Design review of the part built by this model. Coordinates are the model's own, in mm. Face numbers are marked on the shaded views. A direction names the side the tool comes from. Coordinates: 2 decimals unless noted, no trailing zeros. Write each loop counter-clockwise with the first axis right and the second up, starting at its lowest first coordinate (ties: lowest second). Pieces come first, ordered by that corner, then holes.
Q1. Insertion check: pin 1 (3 mm diameter, centred on x = -2, z = 25, fed in from +Y); pin 2 (12 mm diameter, centred on y = 17.5, z = 82, fed in from +X); pin 3 (4 mm diameter, centred on y = -12, z = 10, fed in from +X); pin 4 (2 mm diameter, centred on x = 28, y = 29.5, fed in from +Z). Each pin has a flat end and moves straight along its axis. Give the tip position at first contact, or say it passes through.
Q2. Take a section at A-A (z = 69). Give the boundary of the cut face in (x, y).
Q3. Take a section at B-B (y = 2). Give the boundary of the cut face in (x, z).
Q4. Machinability: for the marked faces 4, 5 and 6, which of the approach directions +Z, -Z, +X, -X, +Y, -Y give a long, thin tool a straight path to every point of the face, cutting with its end or side? Answer none if there is none.
Q5. Take a section at D-D (x = 33). Give the boundary of the cut face in (y, z), and give its area (3 significant figures).
Q6. Take a section at C-C (x = 15.5). Give the boundary of the cut face in (y, z), and give its area (3 significant figures).
Q7. Mouldability with a two-part tool opening along X and no side actions: class the marked faces 1, 2 and 3 as pulls with the +X half, pulls with the -X half, needs draft (parallel to the pull), parting line crosses it, or undercut.
Q8. For probe 1 along X at (y, z) = (1, 35); probe 2 along Z at (x, y) = (-25.5, 3.5); probe 3 along X at (y, z) = (5.5, 100.5), list the stretches that pass through material, from the lowest coordinate up.
Autodesk Fusion 360 part; units mm, degrees
sketch "Sketch1" plane through (0, 0, 0) normal (0, 0, 1) x (1, 0, 0)
  circle A0 centre (0, 0) radius 38.1
  circle A1 centre (0, 0) radius 37.1
  line L0 (24.903, -27.5) -> (24.903, 27.5)
  line L1 (26.903, -25.5468) -> (26.903, 25.5468)
  line L2 (26.903, 12.5) -> (28.903, 12.5)
  line L3 (28.903, 12.5) -> (28.903, -12.5)
  line L4 (28.903, -12.5) -> (26.903, -12.5)
  line L5 (26.903, -12.5) -> (26.903, 12.5)
  line L6 (26.903, 14.5) -> (30.903, 14.5)
  line L7 (30.903, 14.5) -> (30.903, 9.5)
  line L8 (30.903, 9.5) -> (28.903, 9.5)
  line L9 (26.903, -14.5) -> (30.903, -14.5)
  line L10 (30.903, -14.5) -> (30.903, -9.5)
  line L11 (30.903, -9.5) -> (28.903, -9.5)
  line L12 (1.75, 0) -> (22.5, 0)
  line L13 (24.903, 26.75) -> (22.903, 26.75)
  line L14 (22.903, 26.75) -> (22.903, -26.75)
  line L15 (22.903, -26.75) -> (24.903, -26.75)
  line L16 (24.903, -26.75) -> (24.903, 26.75)
  line L17 (22.903, 18.08) -> (11.903, 18.08)
  line L18 (11.903, 18.08) -> (11.903, 5.58)
  line L19 (11.903, 5.58) -> (22.903, 5.58)
  line L20 (22.903, 5.58) -> (22.903, 18.08)
  line L21 (22.903, -13.25) -> (11.903, -13.25)
  line L22 (11.903, -13.25) -> (11.903, -22.5)
  line L23 (11.903, -22.5) -> (22.903, -22.5)
  line L24 (22.903, -22.5) -> (22.903, -13.25)
  line L25 (30.903, -9.5) -> (30.903, 9.5)
  line L26 (0, -38.1) -> (0, 38.1) construction
  line L27 (-38.1, 0) -> (38.1, 0) construction
  line L28 (26.9408, -26.9408) -> (-26.9408, 26.9408) construction
  line L29 (26.9408, 26.9408) -> (-26.9408, -26.9408) construction
  line L30 (0, 37.1) -> (0, 38.1)
  line L31 (-26.2337, 26.2337) -> (-26.9408, 26.9408)
  line L32 (-37.1, 0) -> (-38.1, 0)
  line L33 (-26.9408, -26.9408) -> (-26.2337, -26.2337)
  line L34 (0, -38.1) -> (0, -37.1)
  line L35 (26.9408, -26.9408) -> (26.2337, -26.2337)
  line L36 (38.1, 0) -> (37.1, 0)
  line L37 (26.9408, 26.9408) -> (26.2337, 26.2337)
  line L38 (20.903, 30.6508) -> (20.903, 20.08)
  line L39 (20.903, 20.08) -> (9.903, 20.08)
  line L40 (9.903, 20.08) -> (9.903, 3.58)
  line L41 (9.903, 3.58) -> (22.903, 3.58)
  point P0 (28.903, 0)
  point P1 (22.903, 0)
  dimension "d1" = 76.2
  dimension "d2" = 1
  dimension "d3" = 55
  dimension "d4" = 2
  dimension "d5" = 2
  dimension "d6" = 2
  dimension "d7" = 2
  dimension "d8" = 3
  dimension "d9" = 25
  dimension "d10" = 2
  dimension "d11" = 2
  dimension "d12" = 53.5
  dimension "d13" = 12.5
  dimension "d14" = 11
  dimension "d15" = 8.67
  dimension "d16" = 9.25
  dimension "d17" = 11
  dimension "d18" = 4.25
  dimension "d23" = 45
  dimension "d27" = 2
  dimension "d28" = 2
  dimension "d29" = 2
  dimension "d30" = 2
extrude "Extrude1" add sketch "Sketch1" along normal blind 2 contours A1 L1 L6 L7 L9 L10 L25 | A1 L0 L14 L15 L21 L22 L23 L38 L39 L40 L41 | A1 L0 L13 L14 L17 L18 L19 L38 L39 L40 L41 | L0 L13 L14 L15 L16 L20 L24 makes body 1 at (-3.5853, -7.0522, 0) makes body 2 at (32.7043, -2.5435, 0)
extrude "Extrude2" add sketch "Sketch1" along normal blind 15 contours L1 L2 L3 L6 L7 L8 | L1 L3 L4 L9 L10 L11 bodies 2
extrude "Extrude3" add sketch "Sketch1" along normal blind 120 contours A0 A1 L35 L36 | A0 A1 L30 L37 | A1 L0 L1 L5 L16 | A0 A1 L33 L34 | A0 A1 L31 L32 bodies 2 1
extrude "Extrude4" add sketch "Sketch1" along normal blind 10 contours A1 L0 L13 L14 L17 L18 L19 L38 L39 L40 L41 bodies 2
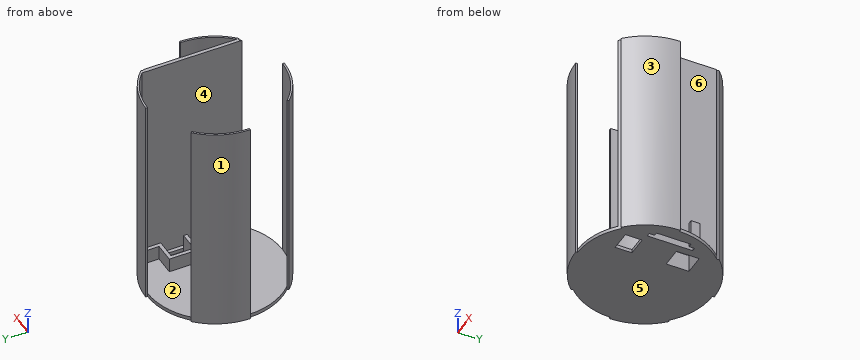
Response:
1. pin 1: stops at y = -36.93
1. pin 2: stops at x = 26.9
1. pin 3: stops at x = 36.76
1. pin 4: passes through
2. outline: (-38.1, 0) - (-37.1, 0) arc R37.1 cw to (-26.23, 26.23) - (-26.94, 26.94) arc R38.1 ccw to start; (-26.94, -26.94) arc R38.1 ccw to (0, -38.1) - (0, -37.1) arc R37.1 cw to (-26.23, -26.23) - close; (0, 37.1) arc R37.1 cw to (24.9, 27.5) - (24.9, -27.5) arc R37.1 ccw to (26.23, -26.23) - (26.94, -26.94) arc R38.1 ccw to (38.1, 0) - (37.1, 0) arc R37.1 cw to (26.9, -25.55) - (26.9, 25.55) arc R37.1 ccw to (26.23, 26.23) - (26.94, 26.94) arc R38.1 ccw to (0, 38.1) - close
3. outline: (-38.05, 0) - (26.9, 0) - (26.9, 120) - (24.9, 120) - (24.9, 2) - (-37.05, 2) - (-37.05, 120) - (-38.05, 120) - close; (30.9, 0) - (37.05, 0) - (37.05, 2) - (30.9, 2) - close
4. face 4: +Z, -Y
4. face 5: -Z, +X, -X, +Y, -Y
4. face 6: +Z
5. outline: (-19.04, 0) - (16.95, 0) - (16.95, 2) - (-16.95, 2) - (-16.95, 120) - (-19.04, 120) - close
5. area: 319 mm2
6. outline: (-33.71, 0) - (-22.5, 0) - (-22.5, 2) - (-33.71, 2) - close; (-13.25, 0) - (5.58, 0) - (5.58, 10) - (3.58, 10) - (3.58, 2) - (-13.25, 2) - close; (18.08, 0) - (34.8, 0) - (34.8, 120) - (33.71, 120) - (33.71, 2) - (20.08, 2) - (20.08, 10) - (18.08, 10) - close
6. area: 255 mm2
7. face 1: pulls with the -X half
7. face 2: undercut
7. face 3: pulls with the +X half
8. probe 1: x = -38.09 to -37.09, 24.9 to 26.9
8. probe 2: z = 0 to 2
8. probe 3: x = -37.7 to -36.69, 24.9 to 26.9
